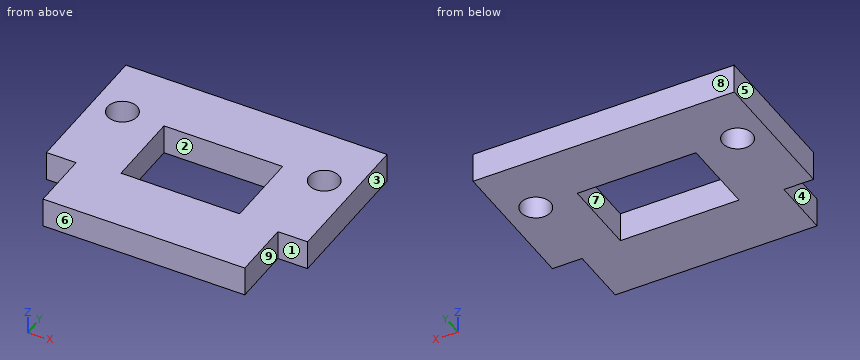
```python
from build123d import *

# Parameters (mm, degrees)
SKETCH1_R           = 1.25
SKETCH1_W           = 10
SKETCH1_H           = 6.5
BOSS_EXTRUDE1_DEPTH = 2.5


with BuildPart() as part:
    # Sketch1 → Boss-Extrude1 (new body)
    with BuildSketch(Plane.XY):
        Polygon((-8.5, -12), (-8.5, -17), (8.5, -17), (8.5, -12), (11, -12), (11, 0), (-11, 0), (-11, -12), align=None)
        with Locations((-8.5, -5)):
            Circle(SKETCH1_R, mode=Mode.SUBTRACT)
        with Locations((8.5, -5)):
            Circle(SKETCH1_R, mode=Mode.SUBTRACT)
        with Locations((0, -8.25)):
            Rectangle(SKETCH1_W, SKETCH1_H, mode=Mode.SUBTRACT)
    extrude(amount=BOSS_EXTRUDE1_DEPTH)


solid = part.part
```
Can you work these out from the model? Positions are in its coordinate system, mm. Face numbers are marked on the shaded views. A direction names the side the tool comes from. Round coordinates to 2 decimals unless told otherwise and drop trailing zeros. Loops run counter-clockwise (first coordinate to the right, second up) from the corner with the lowest first, then second, coordinate; pieces in that order, holes last. Notation, with made-up numbers: M 68,63 L 126,63 A27 ccw 126,85 Z; hole C -21,77 d9. An arc over 180 degrees is marked long. Answer in a Markdown table with one row per item.
1. Please list where these lines run through material, in increasing order: line 1 (Y direction, x = 0, z = 0.65); line 2 (X direction, y = -7, z = 1.7); line 3 (X direction, y = -14, z = 1.5). Write a range as from..to.
Established:
| item | result |
|---|---|
| line 1 | -17..-11.5, -5..0 |
| line 2 | -11..-5, 5..11 |
| line 3 | -8.5..8.5 |
2. On a 3-axis mill with a long thin cutter (end or side, diameter ignored), from which of +Z, -Z, +X, -X, +Y, -Y can I reach the whole of each face in a straight line? I mean the marked faces 1, 2, 3, 4 and 5. Say none if no direction works.
Established:
| item | result |
|---|---|
| face 1 | +Z, -Z, +X, -Y |
| face 2 | +Z, -Z |
| face 3 | +Z, -Z, +X, +Y, -Y |
| face 4 | +Z, -Z, -X, -Y |
| face 5 | +Z, -Z, -X, +Y, -Y |
3. If we section it at B-B, the plane z = 1.1: Please give me the cut outline in (x, y), plus the area to 3 significant figures.
Established:
| item | result |
|---|---|
| outline | M -11,-12 L -8.5,-12 L -8.5,-17 L 8.5,-17 L 8.5,-12 L 11,-12 L 11,0 L -11,0 Z; hole C -8.5,-5 d2.5; hole M -5,-11.5 L 5,-11.5 L 5,-5 L -5,-5 Z; hole C 8.5,-5 d2.5 |
| area | 274 mm² |
4. If we section it at A-A, the plane x = -0.5: Please give me the cut outline in (y, z), plus the area to 4 significant figures.
Established:
| item | result |
|---|---|
| outline | M -17,0 L -11.5,0 L -11.5,2.5 L -17,2.5 Z; M -5,0 L 0,0 L 0,2.5 L -5,2.5 Z |
| area | 26.25 mm² |
5. I'm going to push flat-ended pins straight in: pin 1 Ø1.2 at (y, z) = (-13.5, 0.5) entering from +X; pin 2 Ø1 at (x, y) = (4, -6) entering from -Z; pin 3 Ø3 at (x, y) = (-8.5, -5) entering from -Z; pin 4 Ø0.8 at (x, z) = (-10, 1.5) entering from -Y. Where does each tip first touch, or does it pass through?
Established:
| item | result |
|---|---|
| pin 1 | x = 8.5 |
| pin 2 | through |
| pin 3 | z = 0 |
| pin 4 | y = -12 |
6. Thinking about a two-plate mould opening in Y: for the marked faces 6, 7, 8 and 9, which applies, pulls with the +Y half, pulls with the -Y half, needs draft (parallel to the pull), parting line crosses it, or undercut?
Established:
| item | result |
|---|---|
| face 6 | pulls with the -Y half |
| face 7 | undercut |
| face 8 | pulls with the +Y half |
| face 9 | needs draft |
